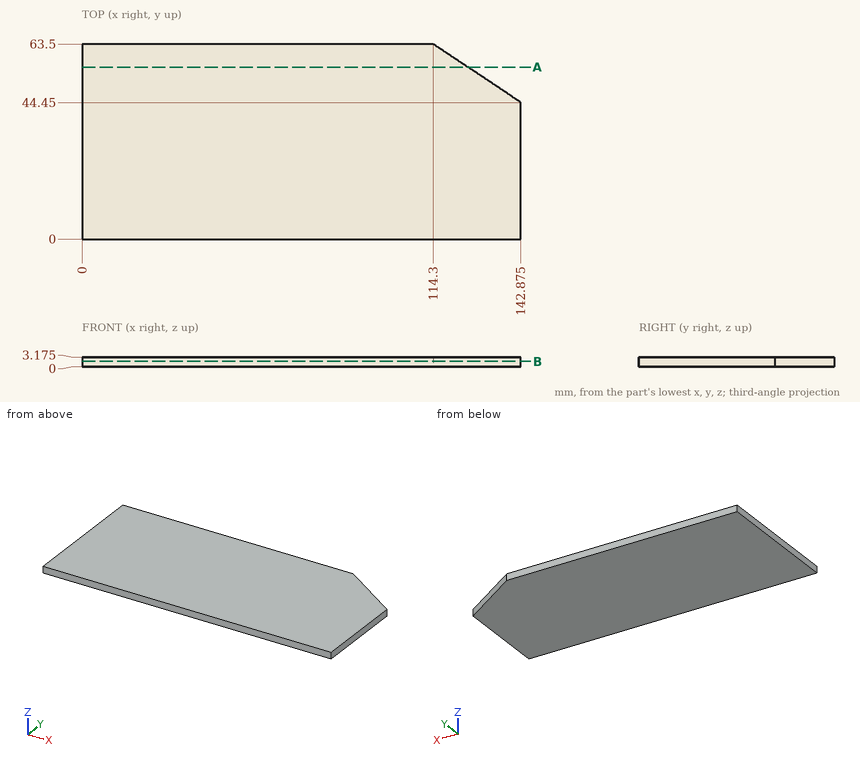
For this review, use the dimensioned drawing (mm, ordinates from the lowest corner) and the shaded views. Give positions to 0.01 mm unless a question says otherwise; leave off trailing zeros. Write each loop counter-clockwise with the first axis right and the second up, starting at its lowest first coordinate (ties: lowest second). Pieces come first, ordered by that corner, then holes. Notation, with made-up numbers: M 43,29.25 L 99,29.25 A16 cw 99,49.25 Z; hole C 69,-14.75 d10. An arc over 180 degrees is marked long. Answer as a JSON object with one key per item and string values. Group by question number.
Item 1: Consider section B-B on z = 1.8. Write out the cut boundary in (x, y) (3 decimals).
Item 2: Consider section A-A on y = 56. Write out the cut boundary in (x, z) (3 decimals).
Item 3: For probe 1 along X at (y, z) = (56, 1); probe 2 along X at (y, z) = (49, 2.4); probe 3 along Y at (x, z) = (135, 2.2), list the stretches that pass through material, from the lowest coordinate up. Write a range as [from, to].
Item 4: For pin 1 Ø1 at (x, y) = (32.5, 49.5) entering from -Z; pin 2 Ø1 at (y, z) = (57, 2.5) entering from +X, all flat-tipped, find the tip position at first contact; note any pin that passes through.
Check result:
{
 "1": {"outline": "M 0,0 L 142.875,0 L 142.875,44.45 L 114.3,63.5 L 0,63.5 Z"},
 "2": {"outline": "M 0,0 L 125.55,0 L 125.55,3.175 L 0,3.175 Z"},
 "3": {"probe 1": "x = [0, 125.55]", "probe 2": "x = [0, 136.05]", "probe 3": "y = [0, 49.7]"},
 "4": {"pin 1": "stops at z = 0", "pin 2": "stops at x = 124.8"}
}
